```python
from build123d import *

# Parameters (mm, degrees)
F1_DEPTH    = 24
F3_W        = 41.439505011
F3_H        = 4
F4_DEPTH    = 25
F5_DEPTH    = 25
F6_DEPTH    = 25
F7_T1_DEPTH = 191.2806862556
F7_T3_DEPTH = 191.2806862556
F8_R        = 5
F9_T1_DEPTH = 48.8746859277
F11_D       = 4.3


# Not quite as in the source:
# - a fillet or chamfer that OpenCascade refuses, or shapes differently, is made with other operations: its cross-section is extruded or revolved along the edge and cut away or added


with BuildPart() as f1:
    # F0 (on Top) → F1 (new body)
    with BuildSketch(Plane.XY):
        with BuildLine():
            ThreePointArc((15, 0), (-3.8035773729, -14.5097484185), (-13.0710398891, 7.3585267695))
            Line((-13.0710398891, 7.3585267695), (-9.4777092406, 21.0662336417))
            Line((-9.4777092406, 21.0662336417), (-13.8306337662, 22.2073068536))
            Line((-13.8306337662, 22.2073068536), (-17.2866620502, 9.0233760402))
            ThreePointArc((-17.2866620502, 9.0233760402), (-3.8959382238, -19.1068486506), (19.439505011, 1.5348110402))
            Line((19.439505011, 1.5348110402), (41.439505011, 1.5348110402))
            Line((41.439505011, 1.5348110402), (41.439505011, 6.0348110402))
            Line((41.439505011, 6.0348110402), (16.5819620065, 6.0348110402))
            Line((16.5819620065, 6.0348110402), (15, 0))
        make_face()
    extrude(amount=F1_DEPTH)

    # F3 (on offset) → F4 (join)
    with BuildSketch(Plane.XZ.offset(19.3651889598)):
        with Locations((20.7197525055, 2)):
            Rectangle(F3_W, F3_H)
        with Locations((20.7197525055, 22)):
            Rectangle(F3_W, F3_H)
    extrude(amount=-F4_DEPTH)

    # F5 (cut): a face of the model
    f5_faces = [f1.faces().sort_by_distance(p)[0] for p in [
        (6.8703868354, -3.2827389678, 20),
    ]]
    extrude(f5_faces, amount=-F5_DEPTH, mode=Mode.SUBTRACT)

    # F6 (cut): a face of the model
    f6_faces = [f1.faces().sort_by_distance(p)[0] for p in [
        (6.8703868354, -3.2827389678, 4),
    ]]
    extrude(f6_faces, amount=-F6_DEPTH, mode=Mode.SUBTRACT)

    # F7: fillet of radius 40.3173664916 on 2 edges, made by hand

    # F7_s2 → F7_t1 (cut)
    with BuildSketch(Plane.XY.offset(-73.6403431278)):
        with BuildLine():
            ThreePointArc((3.9833677598, -19.3651889598), (26.6114599119, -12.4163628374), (41.439505011, 6.0348110402))
            Line((41.439505011, 6.0348110402), (42.188627756, 5.7364637104))
            ThreePointArc((42.188627756, 5.7364637104), (42.2458523408, -6.6651889598), (42.2458523408, -19.3651889598))
            Line((42.2458523408, -19.3651889598), (41.439505011, -20.1715362896))
            Line((41.439505011, -20.1715362896), (3.9833677598, -20.1715362896))
            Line((3.9833677598, -20.1715362896), (3.9833677598, -19.3651889598))
        make_face()
    extrude(amount=F7_T1_DEPTH, mode=Mode.SUBTRACT)

    # F7_s4 → F7_t3 (cut)
    with BuildSketch(Plane.XY.offset(-93.6403431278)):
        with BuildLine():
            ThreePointArc((3.9833677598, -19.3651889598), (26.6114599119, -12.4163628374), (41.439505011, 6.0348110402))
            Line((41.439505011, 6.0348110402), (42.188627756, 5.7364637104))
            ThreePointArc((42.188627756, 5.7364637104), (42.2458523408, -6.6651889598), (42.2458523408, -19.3651889598))
            Line((42.2458523408, -19.3651889598), (41.439505011, -20.1715362896))
            Line((41.439505011, -20.1715362896), (3.9833677598, -20.1715362896))
            Line((3.9833677598, -20.1715362896), (3.9833677598, -19.3651889598))
        make_face()
    extrude(amount=F7_T3_DEPTH, mode=Mode.SUBTRACT)

    # F8
    f8_edges = [f1.edges().sort_by_distance(p)[0] for p in [
        (16.581962, 6.034811, 12),
    ]]
    fillet(f8_edges, radius=F8_R)

    # F9: fillet of radius 5 on 1 edges, made by hand

    # F9_s2 → F9_t1 (cut)
    with BuildSketch(Plane.XY.offset(-12.4373429638)):
        with BuildLine():
            ThreePointArc((-9.4777092406, 21.0662336417), (-12.9919549133, 20.3118564706), (-15.0921376669, 17.394967723))
            Line((-15.0921376669, 17.394967723), (-13.8306337662, 22.2073068536))
            Line((-13.8306337662, 22.2073068536), (-9.4777092406, 21.0662336417))
        make_face()
    extrude(amount=F9_T1_DEPTH, mode=Mode.SUBTRACT)

    # F11 (through all)
    with Locations(Plane.XZ.offset(-1.5348110402)):
        with Locations((30.0100483, 12)):
            Hole(F11_D / 2)


solid = f1.part
```
Geometry check sheet. Reference: the model listing, model coordinates, mm. A direction names the side the tool comes from. Give positions to 0.01 mm unless a question says otherwise; leave off trailing zeros. Order: outer loops, then holes, each group sorted by start corner. A loop starts at its lowest first (then second) coordinate and runs counter-clockwise, first axis right, second up.
1. Section check D-D, the plane x = 18. Enter the section's corners in (y, z).
2. Gauge pin test, flat ends, axial feed: pin 1 Ø1.5 at (y, z) = (1, 11) entering from +X; pin 2 Ø5 at (x, z) = (25.5, 12) entering from -Y; pin 3 Ø4 at (x, z) = (30.01, 12) entering from +Y; pin 4 Ø1.9 at (x, z) = (3, 21) entering from -Y. Record the tip position at first contact, or that the pin passes through.
3. Section check A-A, the plane z = 12. Enter the section's corners in (x, y), and give its area (3 significant figures).
4. Thickness scan on L1, parallel to X at y = 0, z = 18; L2, parallel to X at y = -7, z = 6.5; L3, parallel to Y at x = 33, z = 18.75. Record the ranges inside material, lowest first.
5. Section check C-C, the plane z = 15.5. Enter the section's corners in (x, y).
6. Release check for a two-part mould opening along Z. For faces 1 (the face through (15, -4, 0)), 2 (the face through (25, -7, 4)), 3 (the face through (15.3, 1.14, 12.17)), 4 (the face through (15, -4, 24)) record: pulls with the +Z half, pulls with the -Z half, needs draft (parallel to the pull), parting line crosses it, or undercut.
7. Access from +Z, -Z, +X, -X, +Y, -Y to the whole of each face (thin tool, end or side, straight path). Record for faces 5 (the face through (25, -7, 20)), 6 (the face through (-11.62, -15.66, 11.83)), 7 (the face through (3, -19.365, 22)), 8 (the face through (-11.3, 14.12, 11.83)), 9 (the face through (17.349, 4.965, 12.168)).
8. Section check B-B, the plane y = -1. Enter the section's corners in (x, z).
Values follow:
1. outline: (-16.85, 0) - (5.4, 0) - (5.4, 24) - (-16.85, 24) - (-16.85, 20) - (-7.5, 20) - (-7.5, 4) - (-16.85, 4) - close
2. pin 1: stops at x = 39.43
2. pin 2: stops at y = 1.53
2. pin 3: passes through
2. pin 4: stops at y = -19.39
3. outline: (-17.29, 9.02) arc R19.5 ccw (long way) to (19.44, 1.53) - (27.86, 1.53) - (27.86, 6.03) - (20.44, 6.03) arc R5 ccw to (15.6, 2.3) - (15, 0) arc R15 cw (long way) to (-13.07, 7.36) - (-9.48, 21.07) arc R5 ccw to (-15.09, 17.39) - close; (32.16, 1.53) - (39.32, 1.53) arc R40.32 ccw to (41.44, 6.03) - (32.16, 6.03) - close
3. area: 434 mm2
4. L1: x = -19.5 to -15, 15 to 19.5
4. L2: x = -18.2 to -13.27, 13.27 to 18.2
4. L3: y = 1.53 to 6.03
5. outline: (-17.29, 9.02) arc R19.5 ccw (long way) to (19.44, 1.53) - (39.32, 1.53) arc R40.32 ccw to (41.44, 6.03) - (20.44, 6.03) arc R5 ccw to (15.6, 2.3) - (15, 0) arc R15 cw (long way) to (-13.07, 7.36) - (-9.48, 21.07) arc R5 ccw to (-15.09, 17.39) - close
6. face 1: pulls with the -Z half
6. face 2: undercut
6. face 3: needs draft
6. face 4: pulls with the +Z half
7. face 5: +X, -Y
7. face 6: none
7. face 7: +Z, -Z, +X, -Y
7. face 8: +Z, -Z, +X
7. face 9: +Z, -Z, +Y
8. outline: (-19.47, 0) - (-14.97, 0) - (-14.97, 24) - (-19.47, 24) - close; (14.97, 0) - (37.8, 0) - (37.8, 4) - (19.47, 4) - (19.47, 20) - (37.8, 20) - (37.8, 24) - (14.97, 24) - close
